Could you check a few things on this model? Use its own coordinates, in mm. Face numbers are marked on the shaded views. Round coordinates to 2 decimals unless told otherwise and drop trailing zeros. Write each loop counter-clockwise with the first axis right and the second up, starting at its lowest first coordinate (ties: lowest second). Pieces come first, ordered by that corner, then holes. Notation, with made-up numbers: M 45.25,16.5 L 77.25,16.5 A24 ccw 77.25,42.5 Z; hole C -33.75,71.5 d5. An arc over 180 degrees is marked long. One line per question, with ' | ' between items. Start each with the question number.
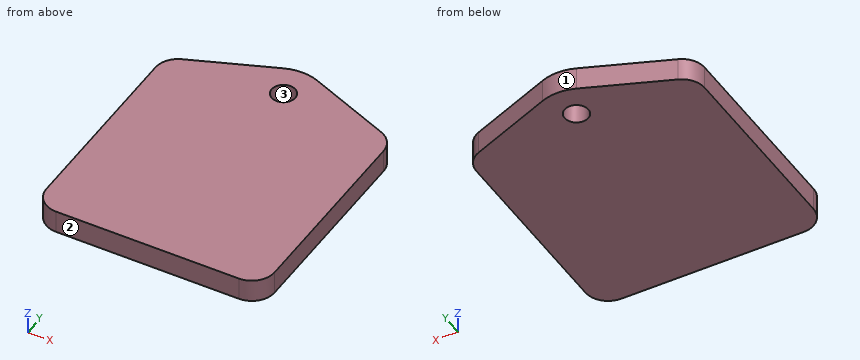
```python
from build123d import *

# Parameters (mm, degrees)
F0_R     = 1.651
F1_DEPTH = 3.175


with BuildPart() as f1:
    # F0 (on Top) → F1 (new body)
    with BuildSketch(Plane.XY):
        with BuildLine():
            ThreePointArc((-15.875, 3.175), (-14.945064, 0.929936), (-12.7, 0))
            Line((-12.7, 0), (12.7, 0))
            ThreePointArc((12.7, 0), (14.945064, 0.929936), (15.875, 3.175))
            Line((15.875, 3.175), (15.875, 29.60042))
            ThreePointArc((15.875, 29.60042), (15.329113, 31.380417), (13.879165, 32.548334))
            Line((13.879165, 32.548334), (2.358331, 37.156668))
            ThreePointArc((2.358331, 37.156668), (0, 37.610841), (-2.358331, 37.156668))
            Line((-2.358331, 37.156668), (-13.879165, 32.548334))
            ThreePointArc((-13.879165, 32.548334), (-15.329113, 31.380417), (-15.875, 29.60042))
            Line((-15.875, 29.60042), (-15.875, 3.175))
        make_face()
        with Locations((0, 33.02)):
            Circle(F0_R, mode=Mode.SUBTRACT)
    extrude(amount=F1_DEPTH)


solid = f1.part
```
1. I'm going to push a flat-ended pin straight in: P1, Ø1.5, axis at x = -2, y = 22.5, coming from the -Z side. Where does the tip first touch, or does it pass through?
2. Suppose I cut it at C-C (z = 0.9). Write out the boundary of the cut face in (x, y) (3 decimals), and give its area (3 significant figures).
3. If we mould it in two halves opening along Y, with no side actions, what happens to the marked faces 1, 2 and 3? For each: released by +Y, released by -Y, zero draft, split by the parting line, or undercut.
4. Suppose I cut it at D-D (x = -6). Write out the boundary of the cut face in (y, z) (3 decimals).
5. Suppose I cut it at B-B (x = 0). Write out the boundary of the cut face in (y, z) (3 decimals).
6. Suppose I cut it at A-A (y = 33.02). Write out the boundary of the cut face in (x, z) (3 decimals), and give its area (3 significant figures).
7. I need wall thicknesses on line 1 along Y through (x, z) = (0, 0.9); line 2 along X through (y, z) = (3, 1.85); line 3 along X through (y, z) = (34.5, 2.45). Which ranges of each line are inside material? Lowest first, please. Write a range as from..to.
Computed:
1) P1: stops at z = 0
2) outline: M -15.875,3.175 A3.175 ccw -12.7,0 L 12.7,0 A3.175 ccw 15.875,3.175 L 15.875,29.6 A3.175 ccw 13.879,32.548 L 2.358,37.157 A6.35 ccw -2.358,37.157 L -13.879,32.548 A3.175 ccw -15.875,29.6 Z; hole C 0,33.02 d3.302 | area: 1,090 mm²
3) face 1: released by +Y | face 2: released by -Y | face 3: undercut
4) outline: M 0,0 L 35.7,0 L 35.7,3.175 L 0,3.175 Z
5) outline: M 0,0 L 31.369,0 L 31.369,3.175 L 0,3.175 Z; M 34.671,0 L 37.611,0 L 37.611,3.175 L 34.671,3.175 Z
6) outline: M -12.7,0 L -1.651,0 L -1.651,3.175 L -12.7,3.175 Z; M 1.651,0 L 12.7,0 L 12.7,3.175 L 1.651,3.175 Z | area: 70.2 mm²
7) line 1: y = 0..31.37, 34.67..37.61 | line 2: x = -15.87..15.87 | line 3: x = -9..-0.73, 0.73..9
